Can you work these out from the drawing? Everything is in mm from the part's minimum corner. A direction names the side the tool comes from. Coordinates: 2 decimals unless noted, no trailing zeros. Order: outer loops, then holes, each group sorted by start corner. A loop starts at its lowest first (then second) coordinate and runs counter-clockwise, first axis right, second up. Notation, with made-up numbers: M 63,64.5 L 70,64.5 A26 cw 70,96.5 Z; hole C 6,31 d9. An arc over 180 degrees is marked long. Answer as a JSON object with one key per item and string values.
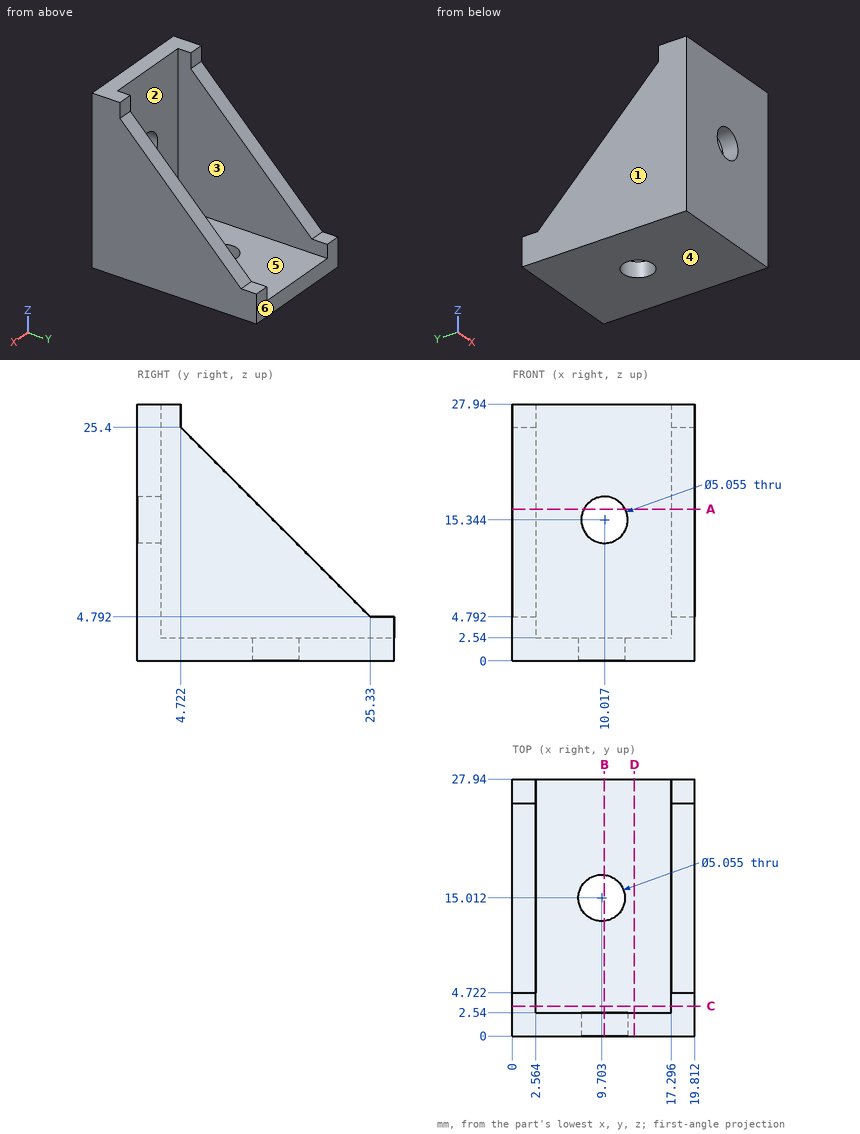
Item 1: Which directions (+Z, -Z, +X, -X, +Y, -Y) give clear straight access to the entire face, cutting with the end or side of a thin tool? Please do the marked faces 5 and 6.
Answers follow:
{"face 5": "+Z, +Y", "face 6": "+Z, -Z, +X, -X, +Y"}
Item 2: If we mould it in two halves opening along X, with no side actions, what happens to the marked faces 1, 2, 3 and 4? For each: pulls with the +X half, pulls with the -X half, needs draft (parallel to the pull), parting line crosses it, or undercut.
Answers follow:
{"face 1": "pulls with the -X half", "face 2": "undercut", "face 3": "undercut", "face 4": "needs draft"}
Item 3: I'm going to push flat-ended pins straight in: pin 1 (6 mm diameter, centred on x = 10.02, z = 15.34, fed in from +Y); pin 2 (3 mm diameter, centred on x = 19, y = 27, fed in from +Z); pin 3 (4.5 mm diameter, centred on x = 9.7, y = 15.01, fed in from +Z); pin 4 (4.5 mm diameter, centred on x = 8, y = 15.5, fed in from +Z). Where does each tip first touch, or does it pass through?
Answers follow:
{"pin 1": "stops at y = 2.54", "pin 2": "stops at z = 4.79", "pin 3": "passes through", "pin 4": "stops at z = 2.54"}
Item 4: I want a section at C-C, the plane y = 3.25. Write out the boundary of the cut face in (x, z) (1 decimal).
Answers follow:
{"outline": "M 0,0 L 19.8,0 L 19.8,27.9 L 17.3,27.9 L 17.3,2.5 L 2.6,2.5 L 2.6,27.9 L 0,27.9 Z"}
Item 5: Please list where these lines run through material, in increasing order: line 1 (X direction, y = 10, z = 11.5) (1 decimal); line 2 (Z direction, x = 6.5, y = 16.5).
Answers follow:
{"line 1": "x = 0 to 2.6, 17.3 to 19.8", "line 2": "z = 0 to 2.54"}
Item 6: I want a section at A-A, the plane z = 16.5. Write out the boundary of the cut face in (x, y) (1 decimal).
Answers follow:
{"outline": "M 0,0 L 7.8,0 L 7.8,2.5 L 2.6,2.5 L 2.6,13.6 L 0,13.6 Z; M 12.3,0 L 19.8,0 L 19.8,13.6 L 17.3,13.6 L 17.3,2.5 L 12.3,2.5 Z"}
Item 7: I want a section at D-D, the plane x = 13.25. Write out the boundary of the cut face in (y, z).
Answers follow:
{"outline": "M 0,0 L 27.94,0 L 27.94,2.54 L 2.54,2.54 L 2.54,27.94 L 0,27.94 Z"}
Item 8: I want a section at B-B, the plane x = 10. Write out the boundary of the cut face in (y, z).
Answers follow:
{"outline": "M 0,0 L 12.5,0 L 12.5,2.54 L 2.54,2.54 L 2.54,12.82 L 0,12.82 Z; M 0,17.87 L 2.54,17.87 L 2.54,27.94 L 0,27.94 Z; M 17.52,0 L 27.94,0 L 27.94,2.54 L 17.52,2.54 Z"}
